Part model, mm, in its own coordinate system. A direction names the side the tool comes from. Give positions to 0.01 mm unless a question says otherwise; leave off trailing zeros. Write each loop counter-clockwise with the first axis right and the second up, starting at its lowest first coordinate (ties: lowest second). Pieces come first, ordered by that corner, then holes. Notation, with made-up numbers: M -12.5,3 L 41.5,3 A30 cw 41.5,28 Z; hole C 64,80 d5. An arc over 180 degrees is marked long. Use a Markdown table: item, result.
```python
from build123d import *

# Parameters (mm, degrees)
SKETCH1_R                                       = 17.5
BOSS_EXTRUDE9_DEPTH                             = 25.5
BOSS_EXTRUDE10_DEPTH                            = 15.4
BOSS_EXTRUDE10_DEPTH_BACK                       = 25.5
CSK_FOR_M3_FLAT_HEAD_MACHINE_SCREW1_D           = 3.6
CSK_FOR_M3_FLAT_HEAD_MACHINE_SCREW1_CSINK_D     = 6.3
CSK_FOR_M3_FLAT_HEAD_MACHINE_SCREW1_CSINK_ANGLE = 90
CSK_FOR_M3_FLAT_HEAD_MACHINE_SCREW2_D           = 3.6
CSK_FOR_M3_FLAT_HEAD_MACHINE_SCREW2_CSINK_D     = 6.3
CSK_FOR_M3_FLAT_HEAD_MACHINE_SCREW2_CSINK_ANGLE = 90
BOSS_EXTRUDE11_DEPTH                            = 15.4


with BuildPart() as part:
    # Sketch1 → Boss-Extrude9 (new body)
    with BuildSketch(Plane.XY):
        with BuildLine():
            ThreePointArc((-19.6, 18.153395679), (0, 37.753395679), (19.6, 18.153395679))
            ThreePointArc((19.6, 18.153395679), (0, -1.446604321), (-19.6, 18.153395679))
        make_face()
        with Locations((0, 18.153395679)):
            Circle(SKETCH1_R, mode=Mode.SUBTRACT)
    extrude(amount=-BOSS_EXTRUDE9_DEPTH)

    # Sketch1<15> → Boss-Extrude10 (add, two sides: drawn at the far end of the back side and taken through both)
    with BuildSketch(Plane.XY.offset(-BOSS_EXTRUDE10_DEPTH_BACK)):
        with BuildLine():
            Line((-23, -1.846604321), (-38, -1.846604321))
            Line((-38, -1.846604321), (-38, -6.846604321))
            Line((-38, -6.846604321), (38, -6.846604321))
            Line((38, -6.846604321), (38, -1.846604321))
            Line((38, -1.846604321), (23, -1.846604321))
            Line((23, -1.846604321), (19.6, 18.153395679))
            ThreePointArc((19.6, 18.153395679), (0, -1.446604321), (-19.6, 18.153395679))
            Line((-19.6, 18.153395679), (-23, -1.846604321))
        make_face()
    extrude(amount=BOSS_EXTRUDE10_DEPTH + BOSS_EXTRUDE10_DEPTH_BACK)

    # CSK for M3 Flat Head Machine Screw1 (through all)
    with Locations(Plane(origin=(0, -1.846604321, 0), x_dir=(1, 0, 0), z_dir=(0, 1, 0))):
        with Locations((-30.5, 15.5), (-30.5, -5.4)):
            CounterSinkHole(CSK_FOR_M3_FLAT_HEAD_MACHINE_SCREW1_D / 2, CSK_FOR_M3_FLAT_HEAD_MACHINE_SCREW1_CSINK_D / 2, counter_sink_angle=CSK_FOR_M3_FLAT_HEAD_MACHINE_SCREW1_CSINK_ANGLE)

    # CSK for M3 Flat Head Machine Screw2 (through all)
    with Locations(Plane(origin=(0, -1.846604321, 0), x_dir=(1, 0, 0), z_dir=(0, 1, 0))):
        with Locations((30.5, -5.4), (30.5, 15.5)):
            CounterSinkHole(CSK_FOR_M3_FLAT_HEAD_MACHINE_SCREW2_D / 2, CSK_FOR_M3_FLAT_HEAD_MACHINE_SCREW2_CSINK_D / 2, counter_sink_angle=CSK_FOR_M3_FLAT_HEAD_MACHINE_SCREW2_CSINK_ANGLE)

    # Sketch1<19> → Boss-Extrude11 (add)
    with BuildSketch(Plane.XY):
        with BuildLine():
            ThreePointArc((-19.6, 18.153395679), (0, -1.446604321), (19.6, 18.153395679))
            Line((19.6, 18.153395679), (17, 18.153395679))
            ThreePointArc((17, 18.153395679), (0, 1.153395679), (-17, 18.153395679))
            Line((-17, 18.153395679), (-19.6, 18.153395679))
        make_face()
    extrude(amount=BOSS_EXTRUDE11_DEPTH)


solid = part.part
```
1. Cut at C-C, the plane x = 0. Give the cut face in (y, z).
Findings below:
| item | result |
|---|---|
| outline | M -6.85,-25.5 L 0.65,-25.5 L 0.65,0 L 1.15,0 L 1.15,15.4 L -6.85,15.4 Z; M 35.65,-25.5 L 37.75,-25.5 L 37.75,0 L 35.65,0 Z |
2. Drill centre lines: L1, parallel to X at y = -4.8, z = 5.4; L2, parallel to Z at x = -30.5, y = -5.9; L3, parallel to Y at x = 0, z = -17. Where is each one in solid material? Low to high.
Findings below:
| item | result |
|---|---|
| L1 | -38 to -32.3, -28.7 to 28.7, 32.3 to 38 |
| L2 | -25.5 to -17.3, -13.7 to 3.6, 7.2 to 15.4 |
| L3 | -6.85 to 0.65, 35.65 to 37.75 |
3. Cut at A-A, the plane z = -15.5. Give the cut face in (x, y).
Findings below:
| item | result |
|---|---|
| outline | M -38,-6.85 L -32.3,-6.85 L -32.3,-3.2 L -33.65,-1.85 L -38,-1.85 Z; M -28.7,-6.85 L 28.7,-6.85 L 28.7,-3.2 L 27.35,-1.85 L 23,-1.85 L 19.6,18.15 A19.6 ccw -19.6,18.15 L -23,-1.85 L -27.35,-1.85 L -28.7,-3.2 Z; M 32.3,-6.85 L 38,-6.85 L 38,-1.85 L 33.65,-1.85 L 32.3,-3.2 Z; hole C 0,18.15 d35 |
4. Two-plate mould, pull along X, no slides. Class faces 1 (the cylindrical face through (-0.43, 37.75, -12.57)), 2 (the flat face through (-18, 18.153, 8)), 3 (the cylindrical face through (-31.468, -5.047, -17.018)), 4 (the flat face through (21.324, 8.013, -5.336)): released by +X, released by -X, zero draft, split by the parting line, or undercut.
Findings below:
| item | result |
|---|---|
| face 1 | split by the parting line |
| face 2 | zero draft |
| face 3 | undercut |
| face 4 | released by +X |
5. Tool access for faces 5 (the cylindrical face through (-3.79, 1.07, -12.57)), 6 (the flat face through (-30, -1.847, -5)), 7 (the flat face through (31, -1.847, -5)): list every direction of +Z, -Z, +X, -X, +Y, -Y with a clear straight run to the whole face (end or side of a thin tool).
Findings below:
| item | result |
|---|---|
| face 5 | -Z |
| face 6 | +Z, -Z, -X, +Y |
| face 7 | +Z, -Z, +X, +Y |
6. Cut at B-B, the plane x = 30.5. Give the cut face in (y, z).
Findings below:
| item | result |
|---|---|
| outline | M -6.85,-25.5 L -1.85,-25.5 L -1.85,-18.65 L -3.2,-17.3 L -6.85,-17.3 Z; M -6.85,-13.7 L -3.2,-13.7 L -1.85,-12.35 L -1.85,2.25 L -3.2,3.6 L -6.85,3.6 Z; M -6.85,7.2 L -3.2,7.2 L -1.85,8.55 L -1.85,15.4 L -6.85,15.4 Z |
7. Cut at D-D, the plane y = 25. Give the cut face in (x, z).
Findings below:
| item | result |
|---|---|
| outline | M -18.37,-25.5 L -16.11,-25.5 L -16.11,0 L -18.37,0 Z; M 16.11,-25.5 L 18.37,-25.5 L 18.37,0 L 16.11,0 Z |
8. Drop flat-ended pins along their axis: P1, Ø3, axis at x = 30.5, z = 5.4, coming from the +Y side; P2, Ø12, axis at y = 18.5, z = -11.5, coming from the +X side; P3, Ø10, axis at x = 26, y = 9.5, coming from the -Z side; P4, Ø3, axis at x = -18, z = 8, coming from the +Y side. Give the stop position or say it passes through.
Findings below:
| item | result |
|---|---|
| P1 | through |
| P2 | x = 20.56 |
| P3 | z = -25.5 |
| P4 | y = 18.15 |
